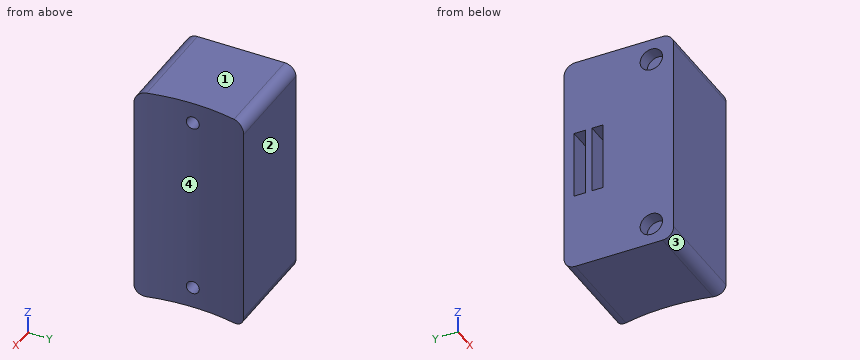
```python
from build123d import *

# Parameters (mm, degrees)
SKETCH_1_W          = 49.5
SKETCH_1_H          = 24.5
EXTRUDE_1_DEPTH     = 22.5
SKETCH_2_R          = 2.5
CUT_EXTRUDE_1_DEPTH = 3
SKETCH_3_W          = 15.2
SKETCH_3_H          = 2.5
CUT_EXTRUDE_2_DEPTH = 8
CUT_EXTRUDE_3_DEPTH = 50
CUT_EXTRUDE_START   = 22.5
SKETCH_5_R          = 1.45
CUT_EXTRUDE_4_DEPTH = 10
FILLET_1_R          = 2.5


with BuildPart() as part:
    # Эскиз1 → Бобышка-Вытянуть1 (new body)
    with BuildSketch(Plane(origin=(0, 0, 0), x_dir=(0, 0, -1), z_dir=(1, 0, 0))):
        Rectangle(SKETCH_1_W, SKETCH_1_H)
    extrude(amount=EXTRUDE_1_DEPTH)

    # Эскиз2 → Вырез-Вытянуть1 (cut)
    with BuildSketch(Plane.ZY):
        with Locations((-20, -7.25)):
            Circle(SKETCH_2_R)
        with Locations((20, -7.25)):
            Circle(SKETCH_2_R)
    extrude(amount=-CUT_EXTRUDE_1_DEPTH, mode=Mode.SUBTRACT)

    # Эскиз3 → Вырез-Вытянуть2 (cut)
    with BuildSketch(Plane.ZY):
        with Locations((0, 4.75)):
            Rectangle(SKETCH_3_W, SKETCH_3_H)
        with Locations((0, 8.75)):
            Rectangle(SKETCH_3_W, SKETCH_3_H)
    extrude(amount=-CUT_EXTRUDE_2_DEPTH, mode=Mode.SUBTRACT)

    # Эскиз4 → Вырез-Вытянуть3 (cut)
    with BuildSketch(Plane(origin=(0, 0, -24.75), x_dir=(-1, 0, 0), z_dir=(0, 0, -1))):
        with BuildLine():
            Line((-22.5, 12.25), (-22.5, -12.25))
            ThreePointArc((-22.5, -12.25), (-20.800548495, 0), (-22.5, 12.25))
        make_face()
    extrude(amount=-CUT_EXTRUDE_3_DEPTH, mode=Mode.SUBTRACT)

    # Эскиз5 → Вырез-Вытянуть4 (cut)
    with BuildSketch(Plane(origin=(0, 0, 0), x_dir=(0, 0, -1), z_dir=(1, 0, 0)).offset(CUT_EXTRUDE_START)):
        with Locations((-20, 0)):
            Circle(SKETCH_5_R)
        with Locations((20, 0)):
            Circle(SKETCH_5_R)
    extrude(amount=-CUT_EXTRUDE_4_DEPTH, mode=Mode.SUBTRACT)

    # Скругление1
    fillet_1_edges = [part.edges().sort_by_distance(p)[0] for p in [
        (11.25, 12.25, -24.75),
        (11.25, -12.25, -24.75),
        (11.25, -12.25, 24.75),
        (11.25, 12.25, 24.75),
    ]]
    fillet(fillet_1_edges, radius=FILLET_1_R)


solid = part.part
```
Can you work these out from the model? Positions are in its coordinate system, mm. Face numbers are marked on the shaded views. Give positions to 0.01 mm unless a question says otherwise; leave off trailing zeros. Write each loop counter-clockwise with the first axis right and the second up, starting at its lowest first coordinate (ties: lowest second). Pieces come first, ordered by that corner, then holes. Notation, with made-up numbers: (-19, -8) - (9, -8) arc R21 cw to (9, 10) - close; hole circle Ø9 at (58, 9.5). An arc over 180 degrees is marked (long way). Write item = value, one per line. Start each with the question number.
1. Please list where these lines run through material, in increasing order: line 1 (Y direction, x = 4.5, z = -7.5); line 2 (Z direction, x = 15.25, y = 0); line 3 (Y direction, x = 1.75, z = -20).
2. Imagine slicing it at A-A (x = 15.5). Please give me the cut outline in (y, z), and give its area (3 significant figures).
3. Imagine slicing it at D-D (x = 2). Please give me the cut outline in (y, z).
4. Imagine slicing it at C-C (y = 0). Please give me the cut outline in (x, z).
5. Imagine slicing it at B-B (z = -20). Please give me the cut outline in (x, y).
6. For pin 1 (3 mm diameter, centred on y = -0.5, z = -13, fed in from -X); pin 2 (1.2 mm diameter, centred on y = 9, z = 3.5, fed in from -X); pin 3 (8 mm diameter, centred on y = -5, z = -11, fed in from +X); pin 4 (8 mm diameter, centred on y = -7.25, z = 20, fed in from +X), each with a flat end and sliding along its axis, tell me the tip position at first contact or that it passes through.
7. Thinking about a two-plate mould opening in Y: for the marked faces 1, 2, 3 and 4, which applies, released by +Y, released by -Y, zero draft, split by the parting line, or undercut?
Worked answers:
q1.line_1 = -12.25 to 3.5, 6 to 7.5, 10 to 12.25
q1.line_2 = -24.75 to -21.45, -18.55 to 18.55, 21.45 to 24.75
q1.line_3 = -12.25 to -9.75, -4.75 to 12.25
q2.outline = (-12.25, -22.25) arc R2.5 ccw to (-9.75, -24.75) - (9.75, -24.75) arc R2.5 ccw to (12.25, -22.25) - (12.25, 22.25) arc R2.5 ccw to (9.75, 24.75) - (-9.75, 24.75) arc R2.5 ccw to (-12.25, 22.25) - close; hole circle Ø2.9 at (0, -20); hole circle Ø2.9 at (0, 20)
q2.area = 1,190 mm2
q3.outline = (-12.25, -22.25) arc R2.5 ccw to (-9.75, -24.75) - (9.75, -24.75) arc R2.5 ccw to (12.25, -22.25) - (12.25, 22.25) arc R2.5 ccw to (9.75, 24.75) - (-9.75, 24.75) arc R2.5 ccw to (-12.25, 22.25) - close; hole circle Ø5 at (-7.25, -20); hole circle Ø5 at (-7.25, 20); hole (3.5, -7.6) - (6, -7.6) - (6, 7.6) - (3.5, 7.6) - close; hole (7.5, -7.6) - (10, -7.6) - (10, 7.6) - (7.5, 7.6) - close
q4.outline = (0, -24.75) - (20.8, -24.75) - (20.8, -21.45) - (12.5, -21.45) - (12.5, -18.55) - (20.8, -18.55) - (20.8, 18.55) - (12.5, 18.55) - (12.5, 21.45) - (20.8, 21.45) - (20.8, 24.75) - (0, 24.75) - close
q5.outline = (0, -12.25) - (22.5, -12.25) arc R45 cw to (20.82, -1.45) - (12.5, -1.45) - (12.5, 1.45) - (20.82, 1.45) arc R45 cw to (22.5, 12.25) - (0, 12.25) - (0, -4.75) - (3, -4.75) - (3, -9.75) - (0, -9.75) - close
q6.pin_1 = 0
q6.pin_2 = 8
q6.pin_3 = 21.71
q6.pin_4 = 22.23
q7.face_1 = zero draft
q7.face_2 = released by +Y
q7.face_3 = released by -Y
q7.face_4 = undercut
